Could you check a few things on this drawing? It's one solid part, dimensions in mm from its lowest x, y, z. A direction names the side the tool comes from. Give positions to 0.01 mm unless a question says otherwise; leave off trailing zeros. Loops run counter-clockwise (first coordinate to the right, second up) from the corner with the lowest first, then second, coordinate; pieces in that order, holes last. Notation, with made-up numbers: M 83,28 L 130,28 A29 cw 130,59 Z; hole C -9.75,41 d1. An arc over 180 degrees is marked long. Answer as a JSON object with one key per item and string values.
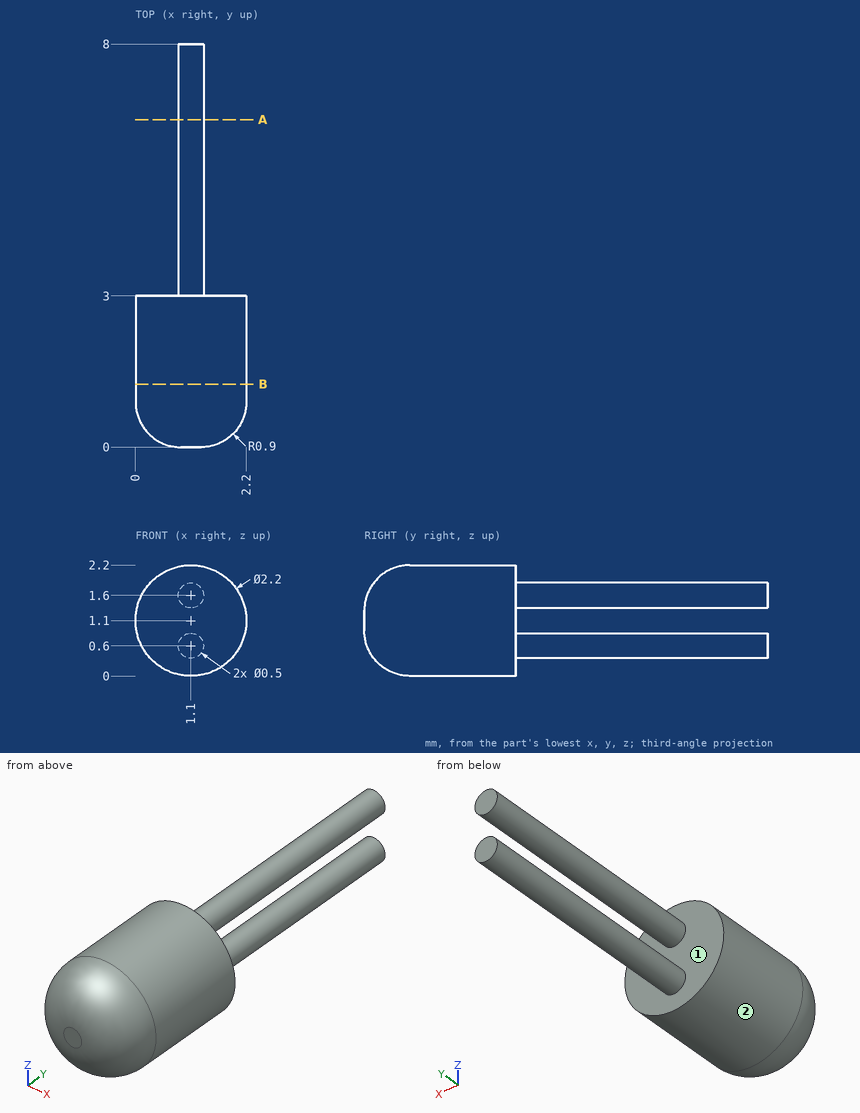
1) For the marked faces 1 and 2, which set-ups out of +Z, -Z, +X, -X, +Y, -Y let a thin tool reach every point of the face, with its end or its side?
Answer list:
{"face 1": "+Y", "face 2": "+Y, -Y"}
2) Please list where these lines run through material, in increasing order: line 1 along X through (y, z) = (4, 1.6); line 2 along Y through (x, z) = (1.8, 1.5); line 3 along X through (y, z) = (0.5, 1.55). Write a range as from..to.
Answer list:
{"line 1": "0.85..1.35", "line 2": "0.23..3", "line 3": "0.2..2"}
3) Suppose I cut it at B-B, the plane y = 1.25. Write out the boundary of the cut face in (x, z).
Answer list:
{"outline": "C 1.1,1.1 d2.2"}
4) Suppose I cut it at A-A, the plane y = 6.5. Write out the boundary of the cut face in (x, z), and give its area (3 significant figures).
Answer list:
{"outline": "C 1.1,0.6 d0.5; C 1.1,1.6 d0.5", "area": "0.393 mm^2"}
